Geometry: final body of the model. Coordinates: model frame, mm. Face numbers are marked on the shaded views. Round coordinates to 2 decimals unless told otherwise and drop trailing zeros. Loops run counter-clockwise (first coordinate to the right, second up) from the corner with the lowest first, then second, coordinate; pieces in that order, holes last. Notation, with made-up numbers: M -20.75,-21 L 13.25,-21 A15 ccw 13.25,0 Z; hole C 15,0.5 d11. An arc over 180 degrees is marked long. Answer as a JSON object with one key per item and string values.
```python
from build123d import *

# Parameters (mm, degrees)
F0_R     = 69.889074
F1_DEPTH = 25
F2_R     = 11.734022
F3_DEPTH = 77


with BuildPart() as f1:
    # F0 (on Front) → F1 (new body)
    with BuildSketch(Plane.XZ):
        with Locations((-15.672464, 14.951888)):
            Circle(F0_R)
    extrude(amount=F1_DEPTH)

    # F2 (on face) → F3 (cut)
    with BuildSketch(Plane.XZ.offset(25)):
        with Locations((-35.751652, 44.561766)):
            Circle(F2_R)
        with Locations((-53.762659, 4.228258)):
            Circle(F2_R)
        with Locations((-20.968921, -25.364967)):
            Circle(F2_R)
        with Locations((17.309731, -3.321078)):
            Circle(F2_R)
        with Locations((8.173501, 39.89602)):
            Circle(F2_R)
    extrude(amount=-F3_DEPTH, mode=Mode.SUBTRACT)


solid = f1.part
```
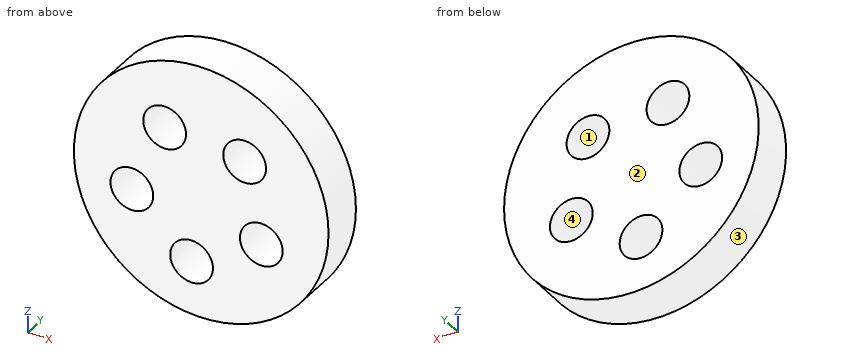
1) Pull-direction query (Z, two-part tool) for the marked faces 1, 2, 3 and 4; classes: +Z half, -Z half, draft (parallel to the pull), parting line (faces both ways), or undercut.
Geometry results:
{"face 1": "undercut", "face 2": "draft", "face 3": "parting line", "face 4": "undercut"}
2) Cut plane D-D on x = 44.5. Return the cut outline in (y, z), and give its area (3 significant figures).
Geometry results:
{"outline": "M -25,-20.6 L 0,-20.6 L 0,50.5 L -25,50.5 Z", "area": "1,780 mm2"}
3) First-contact query: pin 1 (4 mm diameter, centred on y = -5, z = -23.5, fed in from -X); pin 2 (10 mm diameter, centred on x = -7, y = -11, fed in from +Z); pin 3 (4 mm diameter, centred on x = -46.5, y = -10.5, fed in from +Z). Flat tips, straight axial feed; report the tip coordinate or a pass-through.
Geometry results:
{"pin 1": "x = -75.3", "pin 2": "z = 84.74", "pin 3": "z = 78.62"}
4) Cut plane A-A on x = -51. Return the cut outline in (y, z).
Geometry results:
{"outline": "M -25,-45.35 L 0,-45.35 L 0,-7.18 L -25,-7.18 Z; M -25,15.63 L 0,15.63 L 0,75.25 L -25,75.25 Z"}
5) Cut plane B-B on z = -21. Return the cut outline in (x, y).
Geometry results:
{"outline": "M -75.61,-25 L -31.86,-25 L -31.86,0 L -75.61,0 Z; M -10.08,-25 L 44.26,-25 L 44.26,0 L -10.08,0 Z"}
6) Line query: probe 1 along X at (y, z) = (-16.75, 4); probe 2 along Z at (x, y) = (9.5, -21.25); probe 3 along X at (y, z) = (-9.75, 6.5). Output: solid intervals per line, ascending.
Geometry results:
{"probe 1": "-84.7 to -65.49, -42.03 to 8.14, 26.48 to 53.35", "probe 2": "-50.25 to -12.08, 5.44 to 28.24, 51.55 to 80.15", "probe 3": "-85.05 to -65.27, -42.25 to 10.89, 23.73 to 53.7"}
7) Cut plane C-C on y = -5. Return the cut outline in (x, z), and give its area (3 significant figures).
Geometry results:
{"outline": "C -15.67,14.95 d139.78; hole C -53.76,4.23 d23.47; hole C -35.75,44.56 d23.47; hole C -20.97,-25.36 d23.47; hole C 8.17,39.9 d23.47; hole C 17.31,-3.32 d23.47", "area": "13,200 mm2"}
